Source: CAD feature listing. Evaluate the final solid. Frame: model axes, mm. Face numbers are marked on the shaded views. A direction names the side the tool comes from. Give positions to 0.01 mm unless a question says otherwise; leave off trailing zeros. Order: outer loops, then holes, each group sorted by start corner. A loop starts at its lowest first (then second) coordinate and runs counter-clockwise, first axis right, second up. Notation, with made-up numbers: (-4, 9.5) -> (29, 9.5) arc R11 ccw to (29, 20.5) -> close; hole circle Ø5 at (13, 41.5). An arc over 180 degrees is marked (long way). Use one line per item in the form item = value. Start each with the question number.
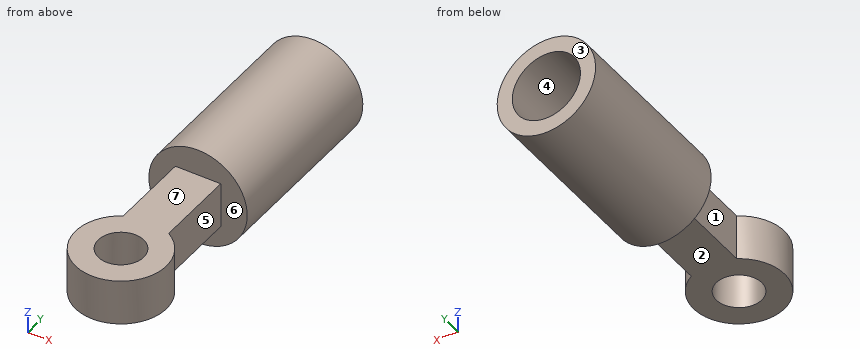
from build123d import *

# Parameters (mm, degrees)
CROQUIS1_R                   = 1.5
SALIENTE_EXTRUIR1_DEPTH      = 3
SALIENTE_EXTRUIR2_DEPTH      = 10
SALIENTE_EXTRUIR2_DEPTH_BACK = 2
CROQUIS2_R                   = 3.25
VACIADO1_START               = 1
VACIADO1_DEPTH               = 1
VACIADO1_START_2             = 9
VACIADO1_2_OUTLINE_R         = 2.25
VACIADO1_2_DEPTH             = 11


with BuildPart() as part:
    # Croquis1 → Saliente-Extruir1 (new body)
    with BuildSketch(Plane.XY):
        with BuildLine():
            Line((1.5, 10), (-1.5, 10))
            Line((-1.5, 10), (-1.5, 2.598076211))
            ThreePointArc((-1.5, 2.598076211), (0, -3), (1.5, 2.598076211))
            Line((1.5, 2.598076211), (1.5, 10))
        make_face()
        Circle(CROQUIS1_R, mode=Mode.SUBTRACT)
    extrude(amount=SALIENTE_EXTRUIR1_DEPTH)

    # Croquis2 → Saliente-Extruir2 (add, two sides: drawn at the far end of the back side and taken through both)
    with BuildSketch(Plane(origin=(0, 10, 0), x_dir=(1, 0, 0), z_dir=(0, 1, 0)).offset(-SALIENTE_EXTRUIR2_DEPTH_BACK)):
        with Locations(Location((0, -1.5, 0), (0, 0, 270))):
            Circle(CROQUIS2_R)
    extrude(amount=SALIENTE_EXTRUIR2_DEPTH + SALIENTE_EXTRUIR2_DEPTH_BACK)

    # Vaciado1: read off the stored shape, not the designer's step
    # Vaciado1 outline → Vaciado1 (cut)
    with BuildSketch(Plane.XY.offset(VACIADO1_START)):
        with BuildLine():
            Line((0.5, 2.449489743), (0.5, 9))
            Line((0.5, 9), (-0.5, 9))
            Line((-0.5, 9), (-0.5, 2.449489743))
            ThreePointArc((-0.5, 2.449489743), (0, 2.5), (0.5, 2.449489743))
        make_face()
    extrude(amount=VACIADO1_DEPTH, mode=Mode.SUBTRACT)

    # Vaciado1 2 outline → Vaciado1 2 (cut)
    with BuildSketch(Plane(origin=(0, 0, 0), x_dir=(1, 0, 0), z_dir=(0, 1, 0)).offset(VACIADO1_START_2)):
        with Locations((0, -1.5)):
            Circle(VACIADO1_2_OUTLINE_R)
    extrude(amount=VACIADO1_2_DEPTH, mode=Mode.SUBTRACT)


solid = part.part
1) Cut plane C-C, the plane y = 13. Return the cut outline in (x, z), plus the area to 3 significant figures.
2) Cut plane B-B, the plane y = 0. Return the cut outline in (x, z).
3) Cut plane D-D, the plane z = 0.5. Return the cut outline in (x, y).
4) Reachability of the marked faces 4, 5, 6 and 7 from +Z, -Z, +X, -X, +Y, -Y: full face, straight path, thin tool, end or side. Return the list, or none.
5) Pin query (flat end, axial travel): pin 1 (2.5 mm diameter, centred on x = 0, y = 0, fed in from +Z); pin 2 (2.5 mm diameter, centred on y = 6, z = 2, fed in from -X); pin 3 (0.5 mm diameter, centred on y = 4.5, z = 1.5, fed in from +X); pin 4 (0.5 mm diameter, centred on x = 0, y = 7, fed in from +Z). Return the tip coordinate at first contact, or that it passes through.
6) Draft query along Y for the marked faces 1, 2 and 3. Return one class per face: +Y half, -Y half, draft (parallel to the pull), parting line (faces both ways), or undercut.
7) Material intervals for probe 1 along X at (y, z) = (13.75, 1.5); probe 2 along Y at (x, z) = (2, -1); probe 3 along X at (y, z) = (14.5, 2.75), sorted ascending.
8) Cut plane A-A, the plane x = 0. Return the cut outline in (y, z), plus the area to 3 significant figures.
Output values:
q1.outline = circle Ø6.5 at (0, 1.5); hole circle Ø4.5 at (0, 1.5)
q1.area = 17.3 mm^2
q2.outline = (-3, 0) -> (-1.5, 0) -> (-1.5, 3) -> (-3, 3) -> close; (1.5, 0) -> (3, 0) -> (3, 3) -> (1.5, 3) -> close
q3.outline = (-3.09, 8) -> (-1.5, 8) -> (-1.5, 2.6) arc R3 ccw (long way) to (1.5, 2.6) -> (1.5, 8) -> (3.09, 8) -> (3.09, 20) -> (2.02, 20) -> (2.02, 9) -> (-2.02, 9) -> (-2.02, 20) -> (-3.09, 20) -> close; hole circle Ø3 at (0, 0)
q4.face_4 = +Y
q4.face_5 = +Z, -Z, +X
q4.face_6 = none
q4.face_7 = +Z, +X, -X, -Y
q5.pin_1 = through
q5.pin_2 = -1.5
q5.pin_3 = 1.5
q5.pin_4 = 3
q6.face_1 = undercut
q6.face_2 = draft
q6.face_3 = +Y half
q7.probe_1 = -3.25 to -2.25, 2.25 to 3.25
q7.probe_2 = 8 to 20
q7.probe_3 = -3 to -1.87, 1.87 to 3
q8.outline = (-3, 0) -> (-1.5, 0) -> (-1.5, 3) -> (-3, 3) -> close; (1.5, 0) -> (8, 0) -> (8, -1.75) -> (20, -1.75) -> (20, -0.75) -> (9, -0.75) -> (9, 1) -> (2.5, 1) -> (2.5, 2) -> (9, 2) -> (9, 3.75) -> (20, 3.75) -> (20, 4.75) -> (8, 4.75) -> (8, 3) -> (1.5, 3) -> close
q8.area = 46.0 mm^2
